from build123d import *

# Parameters (mm, degrees)
SKETCH1_R           = 25.8
SKETCH1_R_2         = 25
BOSS_EXTRUDE1_DEPTH = 7
SKETCH2_R           = 25.8
SKETCH2_R_2         = 21
BOSS_EXTRUDE2_DEPTH = 5
BOSS_EXTRUDE2_TAPER = 26
FILLET3_R           = 10


with BuildPart() as part:
    # Sketch1 → Boss-Extrude1 (new body)
    with BuildSketch(Plane(origin=(0, 0, 0), x_dir=(1, 0, 0), z_dir=(0, 1, 0))):
        with Locations(Location((0, 0, 0), (0, 0, 270))):
            Circle(SKETCH1_R)
        with Locations(Location((0, 0, 0), (0, 0, 270))):
            Circle(SKETCH1_R_2, mode=Mode.SUBTRACT)
    extrude(amount=-BOSS_EXTRUDE1_DEPTH)

    # Sketch2 → Boss-Extrude2 (add)
    with BuildSketch(Plane(origin=(0, 0, 0), x_dir=(1, 0, 0), z_dir=(0, 1, 0))):
        with Locations(Location((0, 0, 0), (0, 0, 270))):
            Circle(SKETCH2_R)
        Circle(SKETCH2_R_2, mode=Mode.SUBTRACT)
    extrude(amount=BOSS_EXTRUDE2_DEPTH, taper=BOSS_EXTRUDE2_TAPER)

    # Fillet3
    fillet3_edges = [part.edges().sort_by_distance(p)[0] for p in [
        (0, 0, -25.8),
    ]]
    fillet(fillet3_edges, radius=FILLET3_R)


solid = part.part
Verification items for the finished model (mm, model axes). A direction names the side the tool comes from. Coordinates: 2 decimals unless noted, no trailing zeros. Write each loop counter-clockwise with the first axis right and the second up, starting at its lowest first coordinate (ties: lowest second). Pieces come first, ordered by that corner, then holes. Notation, with made-up numbers: (-21.5, -28.5) - (12.5, -28.5) arc R6 cw to (12.5, -20.5) - close; hole circle Ø7 at (50, 14.25). An arc over 180 degrees is marked (long way). Answer as a JSON object with one key per item and string values.
(1) Tool access check on faces 1 (the conical face through (-4.58, 0.31, -20.65)), 2 (the flat face through (20.5, 0, -5.7)). Record the directions out of +Z, -Z, +X, -X, +Y, -Y that give a thin tool (end or side, any length) a straight path to the whole face; none if there is none.
Report:
{"face 1": "+Y", "face 2": "-Y"}
(2) Gauge pin test, flat ends, axial feed: pin 1 Ø1 at (x, y) = (16.5, -4.5) entering from +Z; pin 2 Ø4 at (x, z) = (-4.5, -20) entering from +Y; pin 3 Ø6 at (x, z) = (-16, -8) entering from -Y; pin 4 Ø2 at (y, z) = (-2.5, -10) entering from -X. Record the tip position at first contact, or that the pin passes through.
Report:
{"pin 1": "z = 20.24", "pin 2": "y = 3.08", "pin 3": "through", "pin 4": "x = -24.18"}
(3) Thickness scan on line 1 along X through (y, z) = (-2.5, 0); line 2 along X through (y, z) = (-1.25, 13.5); line 3 along Z through (x, y) = (2, -5.5). Record the ranges inside material, lowest first.
Report:
{"line 1": "-25.8 to -25, 25 to 25.8", "line 2": "-21.92 to -21.04, 21.04 to 21.92", "line 3": "-25.72 to -24.92, 24.92 to 25.72"}
(4) Cross-section at A-A on y = -6.25. Record the cut outline in (x, z).
Report:
{"outline": "circle Ø51.6 at (0, 0); hole circle Ø50 at (0, 0)"}
(5) Cross-section at B-B on y = 2.75. Record the cut outline in (x, z), plus the area to 3 significant figures.
Report:
{"outline": "circle Ø48.92 at (0, 0); hole circle Ø44.68 at (0, 0)", "area": "311 mm^2"}
(6) Mould release check, pull along Z, two halves, no side actions. Record for faces 3 (the cylindrical face through (7.75, -4.62, 24.61)), 4 (the cylindrical face through (7.509, -3.451, 23.846)): pulls with the +Z half, pulls with the -Z half, needs draft (parallel to the pull), parting line crosses it, or undercut.
Report:
{"face 3": "parting line crosses it", "face 4": "undercut"}
